Input: part model. Units: mm. Frame: model coordinates. Round coordinates to 2 decimals unless told otherwise and drop trailing zeros. Write each loop counter-clockwise with the first axis right and the second up, starting at its lowest first coordinate (ties: lowest second). Pieces come first, ordered by that corner, then holes. Notation, with made-up numbers: M 89,-13.75 L 127,-13.75 A23 ccw 127,-4.75 Z; hole C -9.75,64.5 d7. An arc over 180 degrees is marked long. Use one line per item in the form item = value. Start each with the question number.
Autodesk Inventor part; units mm, degrees
ref_plane "YZ Plane" through (0, 0, 0) normal (1, 0, 0) x (0, 1, 0)
ref_plane "XZ Plane" through (0, 0, 0) normal (0, 1, 0) x (-1, 0, 0)
ref_plane "XY Plane" through (0, 0, 0) normal (0, 0, 1) x (1, 0, 0)
sketch "Sketch1" plane through (0, 0, 0) normal (0, 0, 1) x (1, 0, 0)
  line L0 (-79.046, 31.5) -> (-62.7751, 31.5)
  line L1 (-62.7751, 28.5) -> (-62.7751, 31.5)
  line L2 (-45.2751, 28.5) -> (-62.7751, 28.5)
  line L3 (-45.2751, 31.5) -> (-45.2751, 28.5)
  line L4 (-45.2751, 31.5) -> (-26.3822, 31.5)
  line L5 (-26.3822, 31.5) -> (-9.5251, 31.5)
  line L6 (-9.5251, 28.5) -> (-9.5251, 31.5)
  line L7 (7.9749, 28.5) -> (-9.5251, 28.5)
  line L8 (7.9749, 31.5) -> (7.9749, 28.5)
  line L9 (7.9749, 31.5) -> (24.8319, 31.5)
  line L10 (24.8319, 31.5) -> (43.4749, 31.5)
  line L11 (43.4749, 28.5) -> (43.4749, 31.5)
  line L12 (60.9749, 28.5) -> (43.4749, 28.5)
  line L13 (60.9749, 31.5) -> (60.9749, 28.5)
  line L14 (60.9749, 31.5) -> (79.046, 31.5)
  circle A0 centre (-73.0751, 8.9448) radius 1.5875
  circle A1 centre (-65.4551, 16.1838) radius 8.115
  circle A2 centre (-42.5951, 16.1838) radius 8.115
  circle A3 centre (-54.0251, 9.5798) radius 2.5
  circle A4 centre (-34.9751, 23.4228) radius 1.5875
  circle A5 centre (33.4249, 8.9448) radius 1.5875
  circle A6 centre (52.4749, 9.5798) radius 2.5
  circle A7 centre (41.0449, 16.1838) radius 8.115
  circle A8 centre (63.9049, 16.1838) radius 8.115
  circle A9 centre (71.5249, 23.4228) radius 1.5875
  circle A10 centre (49.9319, -13.25) radius 3.75
  line L15 (55.4319, -14.25) -> (55.4319, -12.25)
  arc A11 (55.9319, -11.75) -> (55.4319, -12.25) centre (55.9319, -12.25) ccw
  line L16 (55.9319, -11.75) -> (56.9319, -11.75)
  arc A12 (57.4319, -12.25) -> (56.9319, -11.75) centre (56.9319, -12.25) ccw
  line L17 (57.4319, -12.25) -> (57.4319, -14.25)
  arc A13 (56.9319, -14.75) -> (57.4319, -14.25) centre (56.9319, -14.25) ccw
  line L18 (56.9319, -14.75) -> (55.9319, -14.75)
  arc A14 (55.4319, -14.25) -> (55.9319, -14.75) centre (55.9319, -14.25) ccw
  circle A15 centre (-33.176, -14.6) radius 10
  line L19 (-79.046, 31.5) -> (79.046, -31.5) construction
  line L20 (79.046, 31.5) -> (-79.046, -31.5) construction
  line L21 (-8.7519, -31.5) -> (6.2481, -31.5)
  line L22 (-8.7519, -31.5) -> (6.2481, -28.5) construction
  line L23 (6.2481, -31.5) -> (-8.7519, -28.5) construction
  line L24 (-41.2519, -31.5) -> (-26.2519, -31.5)
  line L25 (-73.7519, -31.5) -> (-58.7519, -31.5)
  line L26 (23.7481, -31.5) -> (38.7481, -31.5)
  line L27 (-8.7519, -31.5) -> (6.2481, -31.5)
  line L28 (-41.2519, -31.5) -> (-26.2519, -31.5)
  line L29 (56.2481, -31.5) -> (71.2481, -31.5)
  line L30 (23.7481, -31.5) -> (38.7481, -31.5)
  line L31 (-8.7519, -31.5) -> (6.2481, -31.5)
  line L32 (-58.7519, -31.5) -> (-58.7519, -28.5)
  line L33 (-58.7519, -28.5) -> (-41.2519, -28.5)
  line L34 (-41.2519, -28.5) -> (-41.2519, -31.5)
  line L35 (-26.2519, -31.5) -> (-26.2519, -28.5)
  line L36 (-26.2519, -28.5) -> (-8.7519, -28.5)
  line L37 (-8.7519, -28.5) -> (-8.7519, -31.5)
  line L38 (6.2481, -28.5) -> (23.7481, -28.5)
  line L39 (23.7481, -28.5) -> (23.7481, -31.5)
  line L40 (38.7481, -31.5) -> (38.7481, -28.5)
  line L41 (38.7481, -28.5) -> (56.2481, -28.5)
  line L42 (56.2481, -28.5) -> (56.2481, -31.5)
  line L43 (71.2481, -31.5) -> (71.2481, -28.5)
  line L44 (71.2481, -28.5) -> (79.046, -28.5)
  line L45 (-73.7519, -31.5) -> (-73.7519, -28.5)
  line L46 (-73.7519, -28.5) -> (-79.046, -28.5)
  line L47 (-79.046, 5) -> (-82.046, 5)
  line L48 (-82.046, 5) -> (-82.046, -5)
  line L49 (-82.046, -5) -> (-79.046, -5)
  line L50 (-79.046, 5) -> (-82.046, -5) construction
  line L51 (-82.046, 5) -> (-79.046, -5) construction
  line L52 (0, 0) -> (0, 17) construction
  line L53 (-82.046, 25) -> (-82.046, 15)
  line L54 (-82.046, -15) -> (-82.046, -25)
  line L55 (-82.046, 5) -> (-82.046, -5)
  line L56 (-82.046, 25) -> (-79.046, 25)
  line L57 (-82.046, 15) -> (-79.046, 15)
  line L58 (-82.046, -15) -> (-79.046, -15)
  line L59 (-82.046, -25) -> (-79.046, -25)
  line L60 (-79.046, -25) -> (-79.046, -28.5)
  line L61 (-79.046, -15) -> (-79.046, -5)
  line L62 (-79.046, 5) -> (-79.046, 15)
  line L63 (-79.046, 25) -> (-79.046, 31.5)
  line L64 (79.046, 5) -> (82.046, 5)
  line L65 (82.046, 5) -> (82.046, -5)
  line L66 (82.046, -5) -> (79.046, -5)
  line L67 (79.046, 5) -> (82.046, -5) construction
  line L68 (82.046, 5) -> (79.046, -5) construction
  line L69 (82.046, 25) -> (82.046, 15)
  line L70 (82.046, -15) -> (82.046, -25)
  line L71 (82.046, 5) -> (82.046, -5)
  line L72 (82.046, 25) -> (79.046, 25)
  line L73 (82.046, 15) -> (79.046, 15)
  line L74 (82.046, -15) -> (79.046, -15)
  line L75 (82.046, -25) -> (79.046, -25)
  line L76 (79.046, -25) -> (79.046, -28.5)
  line L77 (79.046, -15) -> (79.046, -5)
  line L78 (79.046, 5) -> (79.046, 15)
  line L79 (79.046, 25) -> (79.046, 31.5)
  line L80 (6.2481, -28.5) -> (6.2481, -31.5)
  point P0 (0, 0)
  point P1 (-1.2519, -30)
  point P2 (-80.546, 0)
  point P3 (80.546, 0)
  dimension "d2" = 20
  dimension "d4" = 15
  dimension "d5" = 3
  dimension "d10" = 32.5
  dimension "d13" = 32.5
  dimension "d17" = 3
  dimension "d18" = 10
  dimension "d21" = 20
  dimension "d24" = 20
extrude "Extrusion1" add sketch "Sketch1" along normal mid plane 3
properties part number "srfsamping"
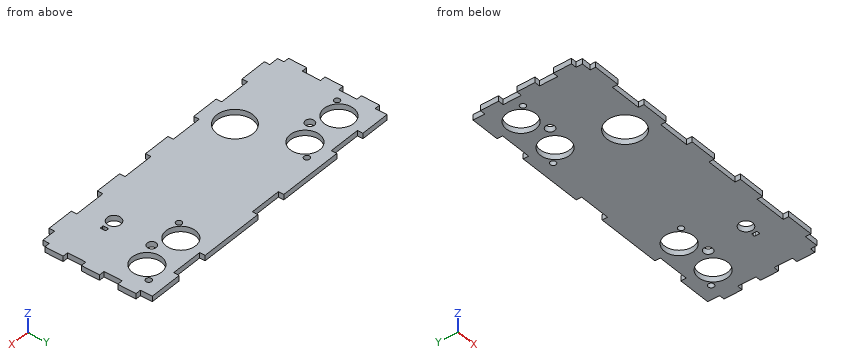
Item 1: Cut plane B-B (x = -39). Output: boundary loops of the cut face in (y, z), plus the area to 3 significant figures.
Item 2: Cut plane C-C (z = 0.55). Give the number of separate pieces and of enclosed holes in the cut face, plus the area to 3 significant figures.
Item 3: Cut plane D-D (x = 15). Output: boundary loops of the cut face in (y, z), plus the area to 3 significant figures.
Item 4: Ray query, line 1 (X direction, y = 15.5, z = -0.85); line 2 (Y direction, x = 49.5, z = -0.1); line 3 (X direction, y = 16.5, z = -1.15). Return the intervals inside material, ascending. Write a range as from..to.
Item 5: Cut plane A-A (y = -7). Output: boundary loops of the cut face in (x, z).
Item 6: First-contact query: pin 1 (1.5 mm diameter, centred on y = 29, z = 0.5, fed in from -X); pin 2 (1.5 mm diameter, centred on y = -30.5, z = -0.5, fed in from -X); pin 3 (1 mm diameter, centred on x = 10, z = -1, fed in from -Y). Flat tips, straight axial feed; report the tip coordinate or a pass-through.
Final values:
q1.outline = M -31.5,-1.5 L -22.73,-1.5 L -22.73,1.5 L -31.5,1.5 Z; M -6.47,-1.5 L 8.91,-1.5 L 8.91,1.5 L -6.47,1.5 Z; M 23.46,-1.5 L 31.5,-1.5 L 31.5,1.5 L 23.46,1.5 Z
q1.area = 96.6 mm^2
q2.separate_pieces = 1
q2.enclosed_holes = 13
q2.area = 8,470 mm^2
q3.outline = M -28.5,-1.5 L 31.5,-1.5 L 31.5,1.5 L -28.5,1.5 Z
q3.area = 180 mm^2
q4.line_1 = -82.05..-73.54, -57.37..-50.68, -34.51..32.96, 49.13..55.82, 71.99..82.05
q4.line_2 = -28.5..-16.98, -9.52..28.5
q4.line_3 = -82.05..-73.56, -57.35..-50.7, -34.49..32.94, 49.15..55.8, 72.01..82.05
q5.outline = M -79.05,-1.5 L -39.68,-1.5 L -39.68,1.5 L -79.05,1.5 Z; M -26.68,-1.5 L 79.05,-1.5 L 79.05,1.5 L -26.68,1.5 Z
q6.pin_1 = -79.05
q6.pin_2 = -73.75
q6.pin_3 = -28.5
